Autodesk Inventor part; units mm, degrees
ref_plane "Work Plane1" through (0, 0, 0) normal (1, 0, 0) x (0, 0, -1)
ref_plane "Work Plane2" through (-0.85, -1.65, 0) normal (0, 0, 1) x (1, 0, 0)
ref_plane "Work Plane3" through (-0.85, -1.65, 0) normal (0, 0, 1) x (1, 0, 0)
ref_plane "Work Plane1" through (0, 0, 0) normal (1, 0, 0) x (0, 0, -1)
sketch "Sketch3" plane through (0, 0, 0) normal (1, 0, 0) x (0, 0, -1)
  circle A0 centre (-3.3861, 0) radius 5.0734
  line L0 (-8.4595, 0) -> (1.6873, 0)
  line L1 (-0.0184, 0) -> (-0.0184, 3.7944)
  point P0 (0, 0)
ref_plane "Work Plane2" through (-0.85, -1.65, 0) normal (0, 0, 1) x (1, 0, 0)
sketch "Sketch5" plane through (-0.85, -1.65, 0) normal (0, 0, 1) x (1, 0, 0)
  line L0 (-0.8, 2.5) -> (0, 3.3)
  line L1 (-0.8, 0.8) -> (-0.8, 2.5)
  line L2 (0, 0) -> (-0.8, 0.8)
  line L3 (2.5, 0) -> (0, 0)
  line L4 (2.5, 3.3) -> (2.5, 0)
  line L5 (0, 3.3) -> (2.5, 3.3)
  circle A0 centre (0.85, 1.65) radius 1.25
revolve "Revolution2" add sketch "Sketch3" angle 360 about axis through (0, 0, 8.4595) along (0, 0, -1) picked at (-5.6014, 0.385) contours L1 L0 A0
ref_plane "Work Plane3" through (-0.85, -1.65, 0) normal (0, 0, 1) x (1, 0, 0)
sketch "Sketch6" plane through (-0.85, -1.65, 0) normal (0, 0, 1) x (1, 0, 0)
  line L0 (0.85, 8.4832) -> (0.85, -5.1832)
  line L1 (-0.8, 2.5) -> (0, 3.3)
  line L2 (-0.8, 0.8) -> (-0.8, 2.5)
  line L3 (0, 0) -> (-0.8, 0.8)
  line L4 (2.5, 0) -> (0, 0)
  line L5 (2.5, 3.3) -> (2.5, 0)
  line L6 (0, 3.3) -> (2.5, 3.3)
  circle A0 centre (0.85, 1.65) radius 1.25
  circle A1 centre (0.85, 1.65) radius 1.25
extrude "Extrusion2" cut sketch "Sketch6" along normal blind 2.5
properties part number "JS5210_hat_top_1"
The model under review builds one solid part; all positions refer to its coordinate system, in mm. Coordinates: 2 decimals unless noted, no trailing zeros. Write each loop counter-clockwise with the first axis right and the second up, starting at its lowest first coordinate (ties: lowest second). Pieces come first, ordered by that corner, then holes. Notation, with made-up numbers: (7, 83.25) - (37, 83.25) arc R18 cw to (37, 96.25) - close; hole circle Ø8 at (-10, 61.5). An arc over 180 degrees is marked (long way). Answer as CSV lines item,"result".
(1) We need section B-B (y = -2). Give the boundary of the cut face in (x, z).
Data:
outline,"(-3.22, 0.02) - (3.22, 0.02) arc R4.66 ccw (long way) to start"
(2) Clearance check with flat-ended pins moving along their axes: pin 1 Ø2 at (x, z) = (0.5, 1) entering from -Y; pin 2 Ø0.8 at (y, z) = (0, 0.5) entering from +X; pin 3 Ø3 at (y, z) = (1.5, 6.5) entering from -X. State where each tip first meets the part, or that it passes through.
Data:
pin 1,"stops at y = -4.87"
pin 2,"stops at x = 4.42"
pin 3,"stops at x = -4.68"
(3) We need section D-D (z = 1.5). Give the boundary of the cut face in (x, y).
Data:
outline,"circle Ø9.42 at (0, 0); hole (-1.65, -0.85) - (-0.85, -1.65) - (1.65, -1.65) - (1.65, 1.65) - (-0.85, 1.65) - (-1.65, 0.85) - close"
(4) We need section A-A (z = 0.5). Give the boundary of the cut face in (x, y), plus the area to 3 significant figures.
Data:
outline,"circle Ø8.35 at (0, 0); hole (-1.65, -0.85) - (-0.85, -1.65) - (1.65, -1.65) - (1.65, 1.65) - (-0.85, 1.65) - (-1.65, 0.85) - close"
area,"44.4 mm2"
(5) For line 1 along X through (y, z) = (1, 1.75); line 2 along Y through (x, z) = (1.5, 0.5); line 3 along X through (y, z) = (-1.5, 1.5), list the stretches that pass through material, from the lowest coordinate up. Write a range as [from, to].
Data:
line 1,"x = [-4.7, -1.5], [1.65, 4.7]"
line 2,"y = [-3.89, -1.65], [1.65, 3.89]"
line 3,"x = [-4.46, -1], [1.65, 4.46]"
(6) We need section C-C (x = -1). Give the boundary of the cut face in (y, z), plus the area to 3 significant figures.
Data:
outline,"(-3.66, 0.02) - (-1.5, 0.02) - (-1.5, 2.5) - (1.5, 2.5) - (1.5, 0.02) - (3.66, 0.02) arc R4.97 ccw (long way) to start"
area,"62.1 mm2"
(7) Mouldability with a two-part tool opening along Y and no side actions: class faces 1 (the flat face through (0, -2, 0.018)), 2 (the flat face through (0, 1.65, 1)) as pulls with the +Y half, pulls with the -Y half, needs draft (parallel to the pull), parting line crosses it, or undercut.
Data:
face 1,"needs draft"
face 2,"undercut"
